Autodesk Fusion 360 part; units mm, degrees
sketch "Sketch1" plane through (0, 0, 0) normal (0, 0, 1) x (1, 0, 0)
  circle A0 centre (-15.1, -12.05) radius 2.15
  circle A1 centre (15.1, -12.05) radius 2.15
  circle A2 centre (-15.1, 12.05) radius 2.15
  circle A3 centre (15.1, 12.05) radius 2.15
  line L0 (-15.5, 16) -> (15.5, 16)
  line L1 (19, 12.5) -> (19, -12.5)
  line L2 (15.5, -16) -> (-15.5, -16)
  line L3 (-19, -12.5) -> (-19, 12.5)
  line L4 (0, 16) -> (0, -16) construction
  line L5 (-19, 3.9253) -> (19, -34.3215) construction
  line L6 (-15.1, 12.05) -> (15.1, 12.05) construction
  line L7 (15.1, 12.05) -> (15.1, -12.05) construction
  line L8 (15.1, -12.05) -> (-15.1, -12.05) construction
  line L9 (-15.1, -12.05) -> (-15.1, 12.05) construction
  circle A4 centre (0, 0) radius 15
  arc A5 (-15.5, 16) -> (-19, 12.5) centre (-15.5, 12.5) ccw
  arc A6 (-19, -12.5) -> (-15.5, -16) centre (-15.5, -12.5) ccw
  arc A7 (15.5, -16) -> (19, -12.5) centre (15.5, -12.5) ccw
  arc A8 (19, 12.5) -> (15.5, 16) centre (15.5, 12.5) ccw
  line L10 (-19, 0) -> (19, 0) construction
  point P0 (-19, 16)
  point P1 (19, 16)
  point P2 (-19, -16)
  point P3 (0, 12.05)
  point P4 (-15.1, 0)
  dimension "d1" = 4.3
  dimension "d4" = 30.2
  dimension "d5" = 24.1
  dimension "d6" = 38
  dimension "d7" = 32
  dimension "d8" = 30
  dimension "d9" = 3.5
extrude "Extrude1" add sketch "Sketch1" along normal blind 1 makes body 1
extrude "Extrude2" add sketch "Sketch1" along normal blind 0.95 contours A4 bodies 1
sketch "Sketch2" plane through (0, 0, 0) normal (0, 0, 1) x (1, 0, 0)
  circle A0 centre (-15.1, -12.05) radius 2.15
  circle A1 centre (15.1, 12.05) radius 2.15
  circle A2 centre (15.1, -12.05) radius 2.15
  circle A3 centre (-15.1, 12.05) radius 2.15
  arc A4 (15.5, -16) -> (19, -12.5) centre (15.5, -12.5) ccw
  line L0 (15.5, -16) -> (-15.5, -16)
  arc A5 (-19, -12.5) -> (-15.5, -16) centre (-15.5, -12.5) ccw
  line L1 (-19, -12.5) -> (-19, 12.5)
  arc A6 (-15.5, 16) -> (-19, 12.5) centre (-15.5, 12.5) ccw
  line L2 (-15.5, 16) -> (15.5, 16)
  arc A7 (19, 12.5) -> (15.5, 16) centre (15.5, 12.5) ccw
  line L3 (19, 12.5) -> (19, -12.5)
  circle A8 centre (0, 0) radius 12.25
  dimension "d14" = 24.5
extrude "Extrude3" add sketch "Sketch2" against normal blind 10 contours A8 bodies 1
ref_plane "WorkPlane1" through (0, 0, 0.5) normal (0, -1, 0) x (1, 0, 0)
sketch "Sketch3" plane through (0, 0, 0) normal (0, -1, 0) x (-1, 0, 0)
  line L0 (12.25, 10) -> (-12.25, 10)
  line L1 (-12.25, 0) -> (12.25, 0)
  circle A0 centre (-12.25, 22.5) radius 12.5
  circle A1 centre (-12.25, 22.5) radius 3.5
  line L2 (-15.61, 21.52) -> (-12.25, 10)
  line L3 (-15.61, 21.52) -> (-8.89, 23.48) construction
  line L4 (-8.89, 23.48) -> (12.25, 10)
  dimension "d17" = 25
  dimension "d18" = 7
  dimension "d19" = 12
extrude "Extrude4" add sketch "Sketch3" along normal mid plane 15 separate body contours A0 A1 L2 L4 | A0 A1 L2 L4 | A1 makes body 2
extrude "Extrude5" add sketch "Sketch3" along normal mid plane 16 contours A1 bodies 2
extrude "Extrude6" add sketch "Sketch3" along normal mid plane 15.8 contours L0 A0 L4 | A0 A1 L2 L4 picked at (-21.2613, 19.5664) bodies 1 2
equation "d4 = 25.9 mm + 4.3 mm"
equation "d5 = 19.8 mm + 4.3 mm"
equation "d20 = ( 15 / 2 ) * 1 mm"
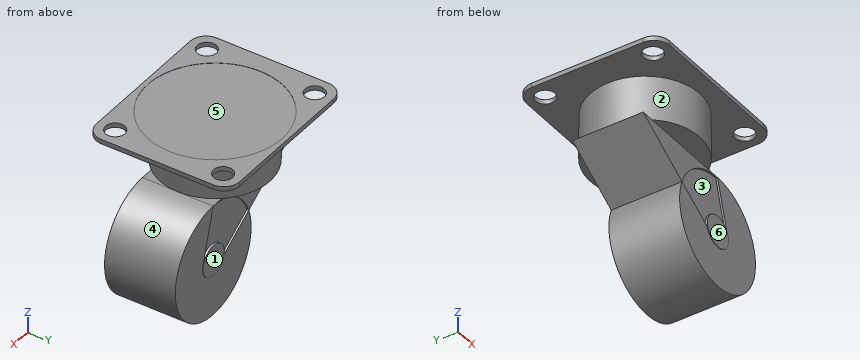
The listing builds one solid part. Answer for the finished solid, in the listing's coordinates (mm). Face numbers are marked on the shaded views. A direction names the side the tool comes from. Round coordinates to 2 decimals unless told otherwise and drop trailing zeros. Write each loop counter-clockwise with the first axis right and the second up, starting at its lowest first coordinate (ties: lowest second). Pieces come first, ordered by that corner, then holes. Notation, with made-up numbers: (25, 73) - (55, 73) arc R16 ccw to (55, 102) - close; hole circle Ø2 at (29.5, -7.5). An arc over 180 degrees is marked (long way). Use a Markdown table: item, result. Add a question column.
1. The part is cut by section A-A (y = 11.5). Write down the section's boundary in (x, z).
2. Flat-ended cylindrical pins translate along their axes: P1, Ø0.9, axis at x = -11, y = 5, coming from the +Z side; P2, Ø2.5, axis at x = -15.1, y = -12.05, coming from the +Z side; P3, Ø1.3, axis at x = -4, y = 11, coming from the -Z side; P4, Ø20, axis at x = 17.5, z = -16.5, coming from the -Y side. Find the tip coordinate at first contact, or state that the pin passes through.
3. The part is cut by section C-C (z = -22.5). Write down the section's boundary in (x, y), and give its area (3 significant figures).
4. For a pull along Z with two mould halves and no side action, classify the marked faces 4, 5 and 6 as +Z half, -Z half, draft (parallel to the pull), parting line (faces both ways), or undercut.
5. The part is cut by section B-B (x = -2.5). Write down the section's boundary in (y, z), and give its area (3 significant figures).
6. A tool of negligible diameter and unlimited length cuts with its end or side. For the marked faces 1, 2 and 3, from which of +Z, -Z, +X, -X, +Y, -Y can it reach the whole face along a straight path? Write none if from no direction.
7. Consider line 1 (Y direction, x = -15.1, z = 0.4); line 2 (Z direction, x = -12.5, y = -6); line 3 (Y direction, x = 8.5, z = -16.5). Determine where each line is inside the solid, lowest interval first.
8. The part is cut by section D-D (y = 3). Write down the section's boundary in (x, z).
Reported:
| question | item | result |
|---|---|---|
| 1 | outline | (-19, 0) - (-17.18, 0) - (-17.18, 1) - (-19, 1) - close; (-13.02, 0) - (-4.22, 0) - (-4.22, -10) - (4.22, -10) - (4.22, 0) - (13.02, 0) - (13.02, 1) - (9.63, 1) - (9.63, 0.95) - (-9.63, 0.95) - (-9.63, 1) - (-13.02, 1) - close; (17.18, 0) - (19, 0) - (19, 1) - (17.18, 1) - close |
| 2 | P1 | z = 0.95 |
| 2 | P2 | through |
| 2 | P3 | z = -10 |
| 2 | P4 | y = -8 |
| 3 | outline | (-0.25, -7.9) - (7.35, -7.9) - (7.35, -7.5) - (8.75, -7.5) - (8.75, -8) - (15.75, -8) - (15.75, -7.9) - (24.75, -7.9) - (24.75, 7.9) - (15.75, 7.9) - (15.75, 8) - (8.75, 8) - (8.75, 7.5) - (7.35, 7.5) - (7.35, 7.9) - (-0.25, 7.9) - close |
| 3 | area | 395 mm^2 |
| 4 | face 4 | undercut |
| 4 | face 5 | +Z half |
| 4 | face 6 | draft |
| 5 | outline | (-16, 0) - (-11.99, 0) - (-11.99, -10) - (-7.9, -10) - (-7.9, -16.22) - (7.9, -16.22) - (7.9, -10) - (11.99, -10) - (11.99, 0) - (16, 0) - (16, 1) - (14.79, 1) - (14.79, 0.95) - (-14.79, 0.95) - (-14.79, 1) - (-16, 1) - close |
| 5 | area | 369 mm^2 |
| 6 | face 1 | -Z, +X, -X, +Y |
| 6 | face 2 | none |
| 6 | face 3 | -Y |
| 7 | line 1 | -16 to -14.2, -9.9 to 9.9, 14.2 to 16 |
| 7 | line 2 | 0 to 0.95 |
| 7 | line 3 | -7.5 to 7.5 |
| 8 | outline | (-19, 0) - (-11.88, 0) - (-11.88, -10) - (-12.25, -10) - (0.53, -18.15) arc R12.5 ccw (long way) to (12.25, -10) - (11.88, -10) - (11.88, 0) - (19, 0) - (19, 1) - (14.7, 1) - (14.7, 0.95) - (-14.7, 0.95) - (-14.7, 1) - (-19, 1) - close |
